from build123d import *

# Parameters (mm, degrees)
F0_W       = 10
F0_H       = 67.7401442081
F0_R       = 1.5
F1_DEPTH   = 2.5
F2_SIZE2   = 1
F2_SIZE    = 5
F2_2_SIZE2 = 1
F2_2_SIZE  = 5


with BuildPart() as f1:
    # F0 (on Top) → F1 (new body, symmetric)
    with BuildSketch(Plane.XY):
        with Locations((-39.6120686829, 11.5640377626)):
            Rectangle(F0_W, F0_H)
        with Locations((-39.6120686829, -18.9060343415)):
            Circle(F0_R, mode=Mode.SUBTRACT)
        with Locations((-39.6120686829, 14.4433356585)):
            Circle(F0_R, mode=Mode.SUBTRACT)
    extrude(amount=F1_DEPTH, both=True)

    # F2
    f2_edges = [f1.edges().sort_by_distance(p)[0] for p in [
        (-44.612069, 45.43411, 0),
    ]]
    f2_side = f1.faces().sort_by_distance((-44.612069, 11.564038, 0))[0]
    chamfer(f2_edges, length=F2_SIZE, length2=F2_SIZE2, reference=f2_side)

    # F2#2
    f2_2_edges = [f1.edges().sort_by_distance(p)[0] for p in [
        (-34.612069, 45.43411, 0),
    ]]
    f2_2_side = f1.faces().sort_by_distance((-34.612069, 11.564038, 0))[0]
    chamfer(f2_2_edges, length=F2_2_SIZE, length2=F2_2_SIZE2, reference=f2_2_side)


solid = f1.part
Geometry: final body of the model. Coordinates: model frame, mm. Round coordinates to 2 decimals unless told otherwise and drop trailing zeros. Loops run counter-clockwise (first coordinate to the right, second up) from the corner with the lowest first, then second, coordinate; pieces in that order, holes last. Notation, with made-up numbers: (88.25, 82) -> (125.25, 82) arc R15 ccw to (125.25, 94) -> close; hole circle Ø2 at (58.5, 27.25). An arc over 180 degrees is marked (long way). One line per question, with ' | ' between items. Start each with the question number.
1. Mould query, pull axis X, two halves, no side actions, for faces 1 (the face through (-38.18, 14.89, -0.04)), 2 (the face through (-44.1, 43, 0)), 3 (the face through (-35.12, 42.97, 0.03)). Classes: pulls with the +X half, pulls with the -X half, needs draft (parallel to the pull), parting line crosses it, or undercut.
2. Section A-A on x = -39.5. Output: boundary loops of the cut face in (y, z).
3. Line query: line 1 along Y through (x, z) = (-40.5, -0.2) (3 decimals); line 2 along X through (y, z) = (42.5, 0.8). Output: solid intervals per line, ascending. Write a range as [from, to].
4. Section B-B on z = 0.4. Output: boundary loops of the cut face in (x, y), and give its area (3 significant figures).
Returned:
1) face 1: undercut | face 2: pulls with the -X half | face 3: pulls with the +X half
2) outline: (-22.31, -2.5) -> (-20.4, -2.5) -> (-20.4, 2.5) -> (-22.31, 2.5) -> close; (-17.41, -2.5) -> (12.95, -2.5) -> (12.95, 2.5) -> (-17.41, 2.5) -> close; (15.94, -2.5) -> (45.43, -2.5) -> (45.43, 2.5) -> (15.94, 2.5) -> close
3) line 1: y = [-22.306, -20.115], [-17.697, 13.234], [15.652, 45.434] | line 2: x = [-44.2, -35.03]
4) outline: (-44.61, -22.31) -> (-34.61, -22.31) -> (-34.61, 40.43) -> (-35.61, 45.43) -> (-43.61, 45.43) -> (-44.61, 40.43) -> close; hole circle Ø3 at (-39.61, -18.91); hole circle Ø3 at (-39.61, 14.44) | area: 658 mm2
